Autodesk Inventor part; units mm, degrees
ref_plane "YZ Plane" through (0, 0, 0) normal (1, 0, 0) x (0, 1, 0)
ref_plane "XZ Plane" through (0, 0, 0) normal (0, 1, 0) x (-1, 0, 0)
ref_plane "XY Plane" through (0, 0, 0) normal (0, 0, 1) x (1, 0, 0)
sketch "Sketch1" plane through (0, 0, 0) normal (0, 1, 0) x (-1, 0, 0)
  line L0 (0, 3.2) -> (-3.2, 3.2)
  line L1 (-3.45, 2.95) -> (-3.45, 1.6)
  arc A0 (-3.45, 1.6) -> (-0.3045, 2.0141) centre (-1.85, 1.6) ccw
  line L2 (0, 0) -> (-5.7029, 0) construction
  line L3 (-1.85, 1.6) -> (-0.3045, 2.0141) construction
  line L4 (0, 2.95) -> (-2.95, 2.95)
  line L5 (-3.2, 2.7) -> (-3.2, 1.6)
  arc A1 (-3.2, 1.6) -> (-0.5038, 1.7019) centre (-1.85, 1.6) ccw
  line L6 (-0.5038, 1.7019) -> (-1.7853, 1.3585) construction
  line L7 (-0.5038, 1.7019) -> (-0.3045, 2.0141)
  line L8 (0, 0) -> (0, 1.4199) construction
  line L9 (0, 3.2) -> (3.2, 3.2)
  line L10 (3.45, 2.95) -> (3.45, 1.6)
  arc A2 (0.3045, 2.0141) -> (3.45, 1.6) centre (1.85, 1.6) ccw
  line L11 (0, 0) -> (5.7029, 0) construction
  line L12 (1.85, 1.6) -> (0.3045, 2.0141) construction
  line L13 (0, 2.95) -> (2.95, 2.95)
  line L14 (3.2, 2.7) -> (3.2, 1.6)
  arc A3 (0.5038, 1.7019) -> (3.2, 1.6) centre (1.85, 1.6) ccw
  line L15 (0.5038, 1.7019) -> (1.7853, 1.3585) construction
  line L16 (0.5038, 1.7019) -> (0.3045, 2.0141)
  arc A4 (-3.2, 3.2) -> (-3.45, 2.95) centre (-3.2, 2.95) ccw
  arc A5 (-2.95, 2.95) -> (-3.2, 2.7) centre (-2.95, 2.7) ccw
  arc A6 (3.2, 2.7) -> (2.95, 2.95) centre (2.95, 2.7) ccw
  arc A7 (3.45, 2.95) -> (3.2, 3.2) centre (3.2, 2.95) ccw
  point P0 (-3.45, 3.2)
  point P1 (-3.2, 2.95)
  point P2 (3.45, 3.2)
  point P3 (3.2, 2.95)
  dimension "d0" = 3.45
  dimension "d1" = 0
  dimension "d2" = 3.2
  dimension "d3" = 15
  dimension "d4" = 1.6
  dimension "d5" = 1.6
  dimension "d6" = 0.25
  dimension "d9" = 0.25
  dimension "d10" = 0.25
  dimension "d11" = 0.25
  dimension "d12" = 0.25
extrude "Extrusion1" add sketch "Sketch1" along normal blind 11.1
sketch "Sketch2" plane through (-3.2, 0, 3.2) normal (0, 0, 1) x (1, 0, 0)
  line L0 (0, 0) -> (6.4, 0)
  line L1 (0, 11.1) -> (6.4, 11.1)
  line L2 (0, 0) -> (0, 11.1)
  line L3 (3.2, 0) -> (3.2, 8.5352) construction
  line L4 (3.2, 3.9) -> (1.67, 3.9)
  line L5 (1.67, 3.9) -> (1.67, 1.67)
  line L6 (1.67, 1.67) -> (0, 0)
  line L7 (-0.25, 0) -> (-0.25, 11.1)
  line L8 (3.2, 3.9) -> (4.73, 3.9)
  line L9 (4.73, 3.9) -> (4.73, 1.67)
  line L10 (4.73, 1.67) -> (6.4, 0)
  dimension "d27" = 7.2
  dimension "d28" = 45
  dimension "d29" = 1.92
  dimension "d30" = 1.53
sketch "Sketch3" plane through (3.45, 0, 2.95) normal (1, 0, 0) x (0, 0, -1)
  line L0 (0, 0) -> (0, 11.1)
  line L1 (6.53, 4.7) -> (1.53, 4.7)
  line L2 (1.53, 4.7) -> (1.53, 1.53)
  line L3 (1.53, 1.53) -> (0, 0)
  line L4 (6.53, 4.7) -> (6.53, -3)
  line L5 (6.53, -3) -> (0, -3)
  line L6 (0, -3) -> (0, 0)
  line L7 (2.95, 11.1) -> (0.9359, 11.1)
  line L8 (-0.25, 0) -> (-0.25, 11.1)
  point P0 (2.95, 0)
  dimension "d13" = 6.4
  dimension "d14" = 1.78
  dimension "d15" = 45
  dimension "d16" = 3
  dimension "d17" = 5
extrude "Extrusion2" cut sketch "Sketch3" against normal through all
sketch "Sketch4" plane through (-0.2602, 4.7, 1.42) normal (0, 0, -1) x (-1, 0, 0)
  line L0 (-1.0096, -4.7) -> (0.4904, -4.7)
  line L1 (0.4904, -4.7) -> (0.4904, 0.8)
  line L2 (0.4904, 0.8) -> (-1.0096, 0.8)
  line L3 (-1.0096, 0.8) -> (-1.0096, -4.7)
  line L4 (-1.0096, -4.7) -> (0.4904, 0.8) construction
  line L5 (0.4904, -4.7) -> (-1.0096, 0.8) construction
  point P0 (-0.2602, -4.7)
  point P1 (-0.2596, -1.95)
  dimension "d20" = 1.5
  dimension "d21" = 0
  dimension "d22" = 5.5
extrude "Extrusion3" cut sketch "Sketch4" along normal blind 11.1 and the other way blind 1
extrude "Extrusion4" cut sketch "Sketch2" against normal through all
equation "\"d4\" = d5"
properties part number "FuseHolder" material "Steel"
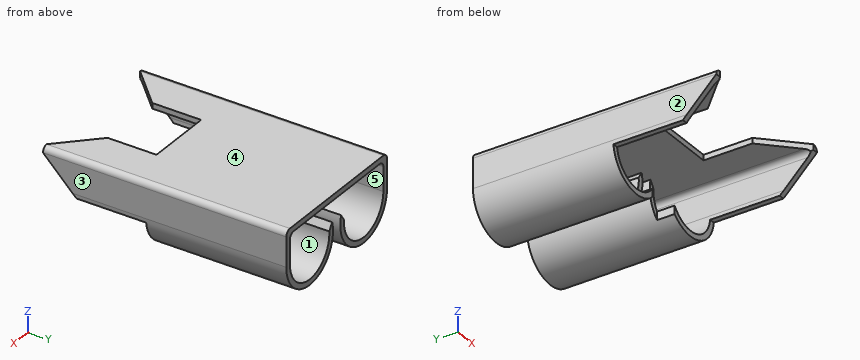
For this review, take the finished solid that the model builds, in its own axes (mm). Face numbers are marked on the shaded views. A direction names the side the tool comes from. Give positions to 0.01 mm unless a question says otherwise; leave off trailing zeros. Loops run counter-clockwise (first coordinate to the right, second up) from the corner with the lowest first, then second, coordinate; pieces in that order, holes last.
Item 1: For line 1 along X through (y, z) = (6.25, 1.8); line 2 along X through (y, z) = (2.75, 2.25); line 3 along Y through (x, z) = (2.5, 0.35), list the stretches that pass through material, from the lowest coordinate up.
Item 2: Take a section at D-D, the plane y = 10. State the section outline as (x, z) points, and give its area (3 significant figures).
Item 3: Insertion check: pin 1 (0.7 mm diameter, centred on x = -1.5, z = 0.5, fed in from -Y); pin 2 (0.5 mm diameter, centred on x = 0.5, z = 1.5, fed in from -Y). Each pin has a flat end and moves straight along its axis. Give the tip position at first contact, or say it passes through.
Item 4: Draft analysis for pull direction X (two halves, no side actions). For the marked faces 3, 4 and 5, state which applies: +X half, -X half, draft (parallel to the pull), parting line (faces both ways), or undercut.
Item 5: Tool access review of the marked faces 1 and 2: name each direction out of +Z, -Z, +X, -X, +Y, -Y from which nothing blocks a thin tool from reaching the whole face with its end or side.
Item 6: Take a section at B-B, the plane y = 2.5. State the section outline as (x, z) points.
Item 7: Take a section at A-A, the plane z = 2.35. State the section outline as (x, y) points, and give its area (3 significant figures).
Item 8: Take a section at C-C, the plane x = -2. State the section outline as (y, z) points.
Calculated:
1. line 1: x = -3.45 to -3.2, -0.44 to -0.26, 0.26 to 0.44, 3.2 to 3.45
1. line 2: x = -3.45 to -3.2, 3.2 to 3.45
1. line 3: y = 4.7 to 11.1
2. outline: (-3.45, 1.6) arc R1.6 ccw (long way) to (-0.3, 2.01) - (-0.5, 1.7) arc R1.35 cw (long way) to (-3.2, 1.6) - (-3.2, 2.7) arc R0.25 cw to (-2.95, 2.95) - (2.95, 2.95) arc R0.25 cw to (3.2, 2.7) - (3.2, 1.6) arc R1.35 cw (long way) to (0.5, 1.7) - (0.3, 2.01) arc R1.6 ccw (long way) to (3.45, 1.6) - (3.45, 2.95) arc R0.25 ccw to (3.2, 3.2) - (-3.2, 3.2) arc R0.25 ccw to (-3.45, 2.95) - close
2. area: 4.85 mm2
3. pin 1: stops at y = 4.7
3. pin 2: stops at y = 5.5
4. face 3: +X half
4. face 4: draft
4. face 5: undercut
5. face 1: +Y, -Y
5. face 2: +Z, -Z, -X, +Y, -Y
6. outline: (-3.45, 1.6) arc R1.6 ccw to (-3.44, 1.42) - (-3.19, 1.42) arc R1.35 cw to (-3.2, 1.6) - (-3.2, 2.7) arc R0.25 cw to (-2.95, 2.95) - (-1.53, 2.95) - (-1.53, 3.2) - (-3.2, 3.2) arc R0.25 ccw to (-3.45, 2.95) - close; (1.53, 2.95) - (2.95, 2.95) arc R0.25 cw to (3.2, 2.7) - (3.2, 1.6) arc R1.35 cw to (3.19, 1.42) - (3.44, 1.42) arc R1.6 ccw to (3.45, 1.6) - (3.45, 2.95) arc R0.25 ccw to (3.2, 3.2) - (1.53, 3.2) - close
7. outline: (-3.45, 0.6) - (-3.2, 0.6) - (-3.2, 11.1) - (-3.45, 11.1) - close; (3.2, 0.6) - (3.45, 0.6) - (3.45, 11.1) - (3.2, 11.1) - close
7. area: 5.25 mm2
8. outline: (1.2, 2.95) - (11.1, 2.95) - (11.1, 3.2) - (1.2, 3.2) - close; (4.7, 0.01) - (11.1, 0.01) - (11.1, 0.26) - (4.7, 0.26) - close
